Source: CAD feature listing. Evaluate the final solid. Frame: model axes, mm. Give positions to 0.01 mm unless a question says otherwise; leave off trailing zeros. Write each loop counter-clockwise with the first axis right and the second up, starting at its lowest first coordinate (ties: lowest second). Pieces come first, ordered by that corner, then holes. Notation, with made-up numbers: (72, 28.25) -> (93, 28.25) arc R12 ccw to (93, 47.25) -> close; hole circle Ø5 at (48, 28.25). An arc over 180 degrees is marked (long way). Write item = value, one per line.
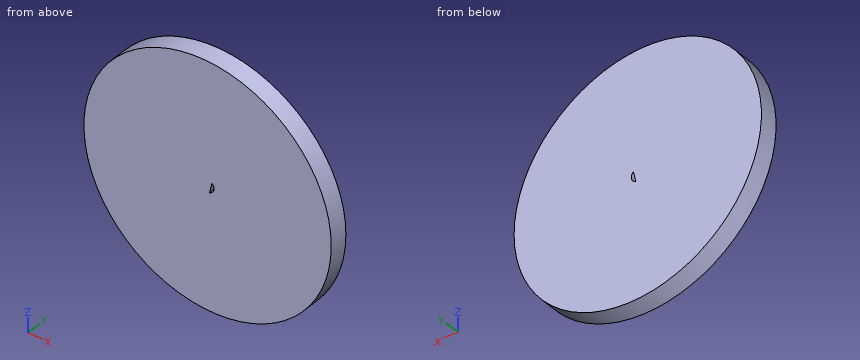
Autodesk Fusion 360 part; units mm, degrees
sketch "Sketch1" plane through (0, 0, 0) normal (0, 1, 0) x (1, 0, 0) in component "wheel"
  circle A0 centre (43.9449, -41.237) radius 67
  circle A1 centre (43.9449, -41.237) radius 3.5
  dimension "d1" = 134
  dimension "d2" = 7
extrude "Extrude1" add sketch "Sketch1" along normal blind 10 in component "wheel"
sketch "Sketch2" plane through (0, 10, 0) normal (0, 1, 0) x (-1, 0, 0) in component "wheel"
  circle A0 centre (-43.9449, 41.237) radius 3.5
  circle A1 centre (-43.9449, 41.237) radius 67
  line L0 (-44.9997, 37.8998) -> (-46.3076, 43.8192)
  dimension "d5" = 1.75
extrude "Extrude2" add sketch "Sketch2" against normal blind 10 contours A0 L0 picked at (-43.9295, 40.8175) in component "wheel"
component "wheel" placed x (1, 0, 0) y (0, 1, 0) z (0, 0, 1) at (0, 0, 0)
1) Cut plane A-A (y = 7.25). Return the cut outline in (x, z).
Computed:
outline = circle Ø134 at (43.94, 41.24); hole (45, 37.9) arc R3.5 ccw to (46.31, 43.82) -> close
2) Contact query for flat-ended pins moving along their axis: pin 1 (1.5 mm diameter, centred on x = -3.5, y = 3.5, fed in from -Z); pin 2 (5 mm diameter, centred on x = 35, y = 8.5, fed in from +Z); pin 3 (6 mm diameter, centred on x = -5.5, y = 1.5, fed in from -Z). Output: stop coordinate, or through.
Computed:
pin_1 = -6.81
pin_2 = 107.93
pin_3 = -7.05
3) Material intervals for L1, parallel to Z at x = 43, y = 7; L2, parallel to X at y = 5.75, z = 41.5 (3 decimals); L3, parallel to X at y = 2, z = 49.5, sorted ascending.
Computed:
L1 = -25.76 to 108.23
L2 = -23.055 to 45.795, 47.435 to 110.944
L3 = -22.54 to 110.43
4) Cut plane C-C (x = 75). Return the cut outline in (y, z).
Computed:
outline = (0, -18.13) -> (10, -18.13) -> (10, 100.61) -> (0, 100.61) -> close
5) Cut plane B-B (z = -9). Return the cut outline in (x, y).
Computed:
outline = (-0.39, 0) -> (88.28, 0) -> (88.28, 10) -> (-0.39, 10) -> close
